Here's how the part is built. I have some questions about the finished solid (model axes, mm). Face numbers are marked on the shaded views. A direction names the side the tool comes from. Coordinates: 2 decimals unless noted, no trailing zeros. Loops run counter-clockwise (first coordinate to the right, second up) from the corner with the lowest first, then second, coordinate; pieces in that order, holes last. Notation, with made-up numbers: (-12, 21.5) - (37, 21.5) arc R23 ccw to (37, 34.5) - close; hole circle Ø4 at (29, 44). An arc over 180 degrees is marked (long way). Use a Markdown table: item, result.
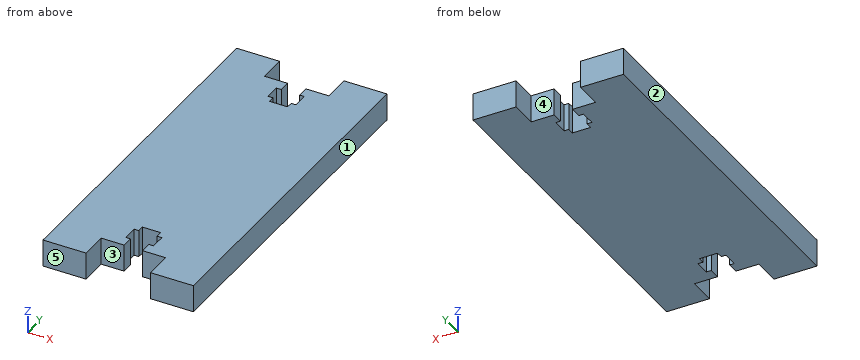
```python
from build123d import *

# Parameters (mm, degrees)
SKETCH1_W           = 20
SKETCH1_H           = 12.7
BOSS_EXTRUDE1_DEPTH = 6.35


with BuildPart() as part:
    # Sketch1 → Boss-Extrude1 (new, symmetric)
    with BuildSketch(Plane.XY):
        Polygon((-35, 68.65), (-35, -68.65), (-15, -68.65), (-4.25, -68.65), (-4.25, -63.35), (-6.5, -63.35), (-6.5, -56.35), (-4.25, -56.35), (-4.25, -53.35), (4.25, -53.35), (4.25, -56.35), (6.5, -56.35), (6.5, -63.35), (4.25, -63.35), (4.25, -68.65), (15, -68.65), (35, -68.65), (35, 68.65), (15, 68.65), (4.25, 68.65), (4.25, 63.35), (6.5, 63.35), (6.5, 56.35), (4.25, 56.35), (4.25, 53.35), (-4.25, 53.35), (-4.25, 56.35), (-6.5, 56.35), (-6.5, 63.35), (-4.25, 63.35), (-4.25, 68.65), (-15, 68.65), align=None)
        with Locations((-25, -75)):
            Rectangle(SKETCH1_W, SKETCH1_H)
        with Locations((25, -75)):
            Rectangle(SKETCH1_W, SKETCH1_H)
        with Locations((25, 75)):
            Rectangle(SKETCH1_W, SKETCH1_H)
        with Locations((-25, 75)):
            Rectangle(SKETCH1_W, SKETCH1_H)
    extrude(amount=BOSS_EXTRUDE1_DEPTH, both=True)


solid = part.part
```
Q1. Please list where these lines run through material, in increasing order: L1, parallel to Y at x = -4.5, z = -5.75; L2, parallel to X at y = 69.5, z = -0.5; L3, parallel to X at y = 57.5, z = -4.5. Write a range as from..to.
Check values:
| item | result |
|---|---|
| L1 | -68.65..-63.35, -56.35..56.35, 63.35..68.65 |
| L2 | -35..-15, 15..35 |
| L3 | -35..-6.5, 6.5..35 |
Q2. If we mould it in two halves opening along X, with no side actions, what happens to the marked faces 1, 2 and 3? For each: pulls with the +X half, pulls with the -X half, needs draft (parallel to the pull), parting line crosses it, or undercut.
Check values:
| item | result |
|---|---|
| face 1 | pulls with the +X half |
| face 2 | pulls with the -X half |
| face 3 | undercut |
Q3. I want a section at A-A, the plane y = -59.5. Write out the boundary of the cut face in (x, z), then the cut area to 3 significant figures.
Check values:
| item | result |
|---|---|
| outline | (-35, -6.35) - (-6.5, -6.35) - (-6.5, 6.35) - (-35, 6.35) - close; (6.5, -6.35) - (35, -6.35) - (35, 6.35) - (6.5, 6.35) - close |
| area | 724 mm^2 |
Q4. Will these pins go through, and if not, where does the flat tip stop? P1, Ø1.8, axis at x = 5, z = 1.5, coming from the -Y side; P2, Ø5.5, axis at x = 10.5, z = -0.5, coming from the +Y side; P3, Ø2, axis at x = -3, z = -3, coming from the -Y side.
Check values:
| item | result |
|---|---|
| P1 | y = -68.65 |
| P2 | y = 68.65 |
| P3 | y = -53.35 |
Q5. Which directions (+Z, -Z, +X, -X, +Y, -Y) give clear straight access to the entire face, cutting with the end or side of a thin tool? Please do the marked faces 4 and 5.
Check values:
| item | result |
|---|---|
| face 4 | +Z, -Z, +Y |
| face 5 | +Z, -Z, +X, -X, -Y |
Q6. I want a section at B-B, the plane x = 9. Write out the boundary of the cut face in (y, z), then the cut area to 3 significant figures.
Check values:
| item | result |
|---|---|
| outline | (-68.65, -6.35) - (68.65, -6.35) - (68.65, 6.35) - (-68.65, 6.35) - close |
| area | 1,740 mm^2 |
